For this review, take the finished solid that the model builds, in its own axes (mm). A direction names the side the tool comes from. Round coordinates to 2 decimals unless told otherwise and drop trailing zeros. Order: outer loops, then holes, each group sorted by start corner. A loop starts at its lowest first (then second) coordinate and runs counter-clockwise, first axis right, second up. Notation, with made-up numbers: M 43,-37 L 97,-37 A32 ccw 97,-4 Z; hole C 7,-29.5 d9. An arc over 180 degrees is marked long. Use a Markdown table: item, result.
from build123d import *

# Parameters (mm, degrees)
F0_W     = 127
F0_H     = 25
F0_W_2   = 12.68
F0_H_2   = 9.89
F1_DEPTH = 1.525
F2_W     = 20
F2_H     = 3
F3_DEPTH = 3.05
F4_W     = 3.1
F4_H     = 4.5
F4_H_2   = 2.5
F4_W_2   = 1.15
F4_H_3   = 3
F5_DEPTH = 3.05
F6_W     = 3.1
F6_H     = 6
F6_R     = 1.575
F7_DEPTH = 3.05
F8_R     = 4


with BuildPart() as f1:
    # F0 (on Front) → F1 (new body, symmetric)
    with BuildSketch(Plane.XZ):
        Rectangle(F0_W, F0_H)
        with Locations((-44.46, 0)):
            Rectangle(F0_W_2, F0_H_2, mode=Mode.SUBTRACT)
        with Locations((44.46, 0)):
            Rectangle(F0_W_2, F0_H_2, mode=Mode.SUBTRACT)
    extrude(amount=F1_DEPTH, both=True)

    # F2 (on face) → F3 (join, through all)
    with BuildSketch(Plane.XZ.offset(1.525)):
        with Locations((-35, 14)):
            Rectangle(F2_W, F2_H)
        with Locations((35, 14)):
            Rectangle(F2_W, F2_H)
    extrude(amount=-F3_DEPTH)

    # F4 (on face) → F5 (cut, through all)
    with BuildSketch(Plane.XZ.offset(1.525)):
        with Locations((0, 10.25)):
            Rectangle(F4_W, F4_H)
        with Locations((0, 6.75)):
            Rectangle(F4_W, F4_H_2)
        with Locations((-2.125, 6.75)):
            Rectangle(F4_W_2, F4_H_2)
        with Locations((2.125, 6.75)):
            Rectangle(F4_W_2, F4_H_2)
        with Locations((0, 4)):
            Rectangle(F4_W, F4_H_3)
    extrude(amount=-F5_DEPTH, mode=Mode.SUBTRACT)

    # F6 (on face) → F7 (cut, through all)
    with BuildSketch(Plane.XZ.offset(1.525)):
        with Locations((-58.05, 7)):
            Rectangle(F6_W, F6_H)
        with Locations((-58.05, -7)):
            Rectangle(F6_W, F6_H)
        with Locations((-58.05, 0)):
            Circle(F6_R)
        with Locations((58.05, 7)):
            Rectangle(F6_W, F6_H)
        with Locations((58.05, -7)):
            Rectangle(F6_W, F6_H)
        with Locations((58.05, 0)):
            Circle(F6_R)
    extrude(amount=-F7_DEPTH, mode=Mode.SUBTRACT)

    # F8
    f8_edges = [f1.edges().sort_by_distance(p)[0] for p in [
        (-63.5, 0, -12.5),
        (63.5, 0, -12.5),
    ]]
    fillet(f8_edges, radius=F8_R)


solid = f1.part
Q1. Machinability: for faces 5 (the flat face through (-1, 1.525, 2)), 6 (the flat face through (44, 0, 4.945)), 7 (the flat face through (-1.55, 0, 10)), which of the approach directions +Z, -Z, +X, -X, +Y, -Y give a long, thin tool a straight path to every point of the face, cutting with its end or side? Answer none if there is none.
Determined:
| item | result |
|---|---|
| face 5 | +Z, -Z, +X, -X, +Y |
| face 6 | +Y, -Y |
| face 7 | +Z, +Y, -Y |
Q2. Add section B-B (x = -49.5). Write out the cut boundary in (y, z) (3 decimals).
Determined:
| item | result |
|---|---|
| outline | M -1.525,-12.5 L 1.525,-12.5 L 1.525,-4.945 L -1.525,-4.945 Z; M -1.525,4.945 L 1.525,4.945 L 1.525,12.5 L -1.525,12.5 Z |
Q3. Add section A-A (z = 6.75). Write out the cut boundary in (x, y) (3 decimals).
Determined:
| item | result |
|---|---|
| outline | M -63.5,-1.525 L -59.6,-1.525 L -59.6,1.525 L -63.5,1.525 Z; M -56.5,-1.525 L -2.7,-1.525 L -2.7,1.525 L -56.5,1.525 Z; M 2.7,-1.525 L 56.5,-1.525 L 56.5,1.525 L 2.7,1.525 Z; M 59.6,-1.525 L 63.5,-1.525 L 63.5,1.525 L 59.6,1.525 Z |
Q4. Add section D-D (y = 0.95). Give the number of separate pieces and of enclosed holes in the cut face, then the cut area to 3 significant figures.
Determined:
| item | result |
|---|---|
| separate pieces | 1 |
| enclosed holes | 8 |
| area | 2,910 mm^2 |
Q5. Wall thickness on line 1 along Z through (x, y) = (-58.05, 0.3) (3 decimals); line 2 along X through (y, z) = (1.1, 5.25); line 3 along X through (y, z) = (-0.8, 3): over which ranges is each line inside the solid? List them lowest first. Write a range as [from, to].
Determined:
| item | result |
|---|---|
| line 1 | z = [-12.5, -10], [-4, -1.575], [1.575, 4], [10, 12.5] |
| line 2 | x = [-63.5, -59.6], [-56.5, -1.55], [1.55, 56.5], [59.6, 63.5] |
| line 3 | x = [-63.5, -50.8], [-38.12, -1.55], [1.55, 38.12], [50.8, 63.5] |
Q6. Add section C-C (z = 0). Write out the cut boundary in (x, y) (3 decimals), then the cut area to 3 significant figures.
Determined:
| item | result |
|---|---|
| outline | M -63.5,-1.525 L -59.625,-1.525 L -59.625,1.525 L -63.5,1.525 Z; M -56.475,-1.525 L -50.8,-1.525 L -50.8,1.525 L -56.475,1.525 Z; M -38.12,-1.525 L 38.12,-1.525 L 38.12,1.525 L -38.12,1.525 Z; M 50.8,-1.525 L 56.475,-1.525 L 56.475,1.525 L 50.8,1.525 Z; M 59.625,-1.525 L 63.5,-1.525 L 63.5,1.525 L 59.625,1.525 Z |
| area | 291 mm^2 |
Q7. Clearance check with flat-ended pins moving along their axes: pin 1 (0.9 mm diameter, centred on x = 2, y = -0.5, fed in from +Z); pin 2 (0.9 mm diameter, centred on x = 0, y = 0, fed in from +Z). State where each tip first meets the part, or that it passes through.
Determined:
| item | result |
|---|---|
| pin 1 | stops at z = 12.5 |
| pin 2 | stops at z = 2.5 |
Q8. Draft analysis for pull direction X (two halves, no side actions). For faces 1 (the flat face through (63.5, 0, 2)), 2 (the flat face through (-54, 0, 12.5)), 3 (the cylindrical face through (-62.359, -0.021, -11.297)), 4 (the flat face through (-56.5, 0, 7)), state which applies: pulls with the +X half, pulls with the -X half, needs draft (parallel to the pull), parting line crosses it, or undercut.
Determined:
| item | result |
|---|---|
| face 1 | pulls with the +X half |
| face 2 | needs draft |
| face 3 | pulls with the -X half |
| face 4 | undercut |
